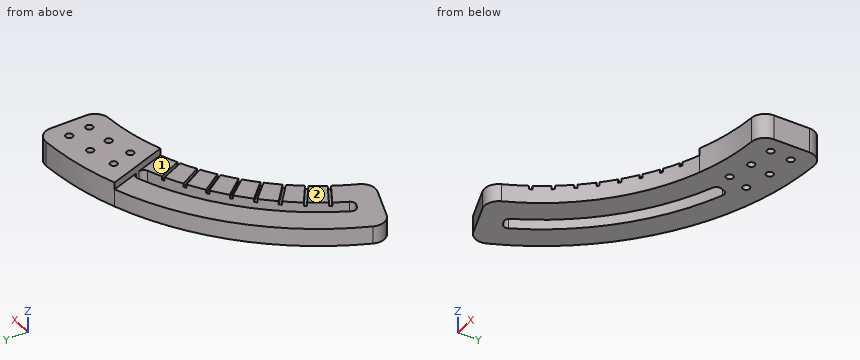
from build123d import *

# Parameters (mm, degrees)
BOSS_EXTRUDE2_DEPTH = 5
SKETCH1_5_R         = 1
BOSS_EXTRUDE3_DEPTH = 7
FILLET1_R           = 1.5
CUT_EXTRUDE1_DEPTH  = 1


with BuildPart() as part:
    # Sketch1 → Boss-Extrude2 (new body)
    with BuildSketch(Plane.XY):
        with BuildLine():
            ThreePointArc((-56.868678478, 24.697234828), (-42.491353844, 45.149583038), (-21.205248886, 58.260942489))
            Line((-21.205248886, 58.260942489), (-23.257369746, 63.899098213))
            Line((-23.257369746, 63.899098213), (-23.599389889, 64.838790834))
            ThreePointArc((-23.599389889, 64.838790834), (-46.615724325, 50.87213624), (-62.535237306, 29.16066006))
            Line((-62.535237306, 29.16066006), (-66.160468454, 30.851133107))
            ThreePointArc((-66.160468454, 30.851133107), (-49.318085156, 53.821245587), (-24.967470463, 68.597561317))
            Line((-24.967470463, 68.597561317), (-25.309490606, 69.537253938))
            Line((-25.309490606, 69.537253938), (-27.361611466, 75.175409663))
            ThreePointArc((-27.361611466, 75.175409663), (-55.059776129, 58.038100009), (-73.631131577, 31.280288725))
            ThreePointArc((-73.631131577, 31.280288725), (-73.618051339, 28.121820986), (-71.317655571, 25.957503806))
            Line((-71.317655571, 25.957503806), (-61.90570605, 22.531834333))
            ThreePointArc((-61.90570605, 22.531834333), (-58.95783549, 22.615790046), (-56.868678478, 24.697234828))
        make_face()
    extrude(amount=BOSS_EXTRUDE2_DEPTH)

    # Sketch1<5> → Boss-Extrude3 (add)
    with BuildSketch(Plane.XY):
        with BuildLine():
            ThreePointArc((-21.205248886, 58.260942489), (-12.61233393, 60.703616308), (-3.757575758, 61.886029315))
            ThreePointArc((-3.757575758, 61.886029315), (-1.087123675, 63.137298701), (0, 65.878676368))
            Line((0, 65.878676368), (0, 75.894663844))
            ThreePointArc((0, 75.894663844), (-1.247011194, 78.796568844), (-4.210526316, 79.889119836))
            ThreePointArc((-4.210526316, 79.889119836), (-15.961038091, 78.39161475), (-27.361611466, 75.175409663))
            Line((-27.361611466, 75.175409663), (-21.205248886, 58.260942489))
        make_face()
        with Locations((-4.594594595, 67.844599641)):
            Circle(SKETCH1_5_R, mode=Mode.SUBTRACT)
        with Locations((-11.808076081, 66.966927205)):
            Circle(SKETCH1_5_R, mode=Mode.SUBTRACT)
        with Locations((-18.886713057, 65.324513545)):
            Circle(SKETCH1_5_R, mode=Mode.SUBTRACT)
        with Locations((-5, 73.830887845)):
            Circle(SKETCH1_5_R, mode=Mode.SUBTRACT)
        with Locations((-12.849965147, 72.875773723)):
            Circle(SKETCH1_5_R, mode=Mode.SUBTRACT)
        with Locations((-20.553187739, 71.088441211)):
            Circle(SKETCH1_5_R, mode=Mode.SUBTRACT)
    extrude(amount=BOSS_EXTRUDE3_DEPTH)

    # Fillet1
    fillet1_edges = [part.edges().sort_by_distance(p)[0] for p in [
        (-66.160468454, 30.851133107, 2.5),
        (-62.535237306, 29.16066006, 2.5),
        (-23.599389889, 64.838790834, 2.5),
        (-24.967470463, 68.597561317, 2.5),
    ]]
    fillet(fillet1_edges, radius=FILLET1_R)

    # Sketch2 → Cut-Extrude1 (cut)
    with BuildSketch(Plane.XY.offset(5)):
        Polygon((-26.182734595, 55.202574904), (-25.457688366, 55.540669514), (-29.670325491, 64.574698983), (-30.395371721, 64.236604373), align=None)
        Polygon((-30.894322803, 52.71053676), (-35.87829712, 61.343033502), (-35.185476797, 61.743033502), (-30.20150248, 53.11053676), align=None)
        Polygon((-35.370786559, 49.817339603), (-41.088167015, 57.982605105), (-40.43284538, 58.441466254), (-34.715464924, 50.276200752), align=None)
        Polygon((-39.578057272, 46.545002412), (-45.985331149, 54.180894073), (-45.372495595, 54.695124161), (-38.965221718, 47.059232499), align=None)
        Polygon((-43.484115072, 42.918429647), (-50.532519147, 49.966833722), (-49.966833722, 50.532519147), (-42.918429647, 43.484115072), align=None)
        Polygon((-47.059232499, 38.965221718), (-54.695124161, 45.372495595), (-54.180894073, 45.985331149), (-46.545002412, 39.578057272), align=None)
        Polygon((-50.276200752, 34.715464924), (-58.441466254, 40.43284538), (-57.982605105, 41.088167015), (-49.817339603, 35.370786559), align=None)
        Polygon((-53.11053676, 30.20150248), (-61.743033502, 35.185476797), (-61.343033502, 35.878297121), (-52.71053676, 30.894322803), align=None)
    extrude(amount=-CUT_EXTRUDE1_DEPTH, mode=Mode.SUBTRACT)


solid = part.part
The model under review builds one solid part; all positions refer to its coordinate system, in mm. Face numbers are marked on the shaded views. A direction names the side the tool comes from. Give positions to 0.01 mm unless a question says otherwise; leave off trailing zeros. Order: outer loops, then holes, each group sorted by start corner. A loop starts at its lowest first (then second) coordinate and runs counter-clockwise, first axis right, second up. Notation, with made-up numbers: M 40.5,62 L 95.5,62 A25 ccw 95.5,88 Z; hole C -37,-12.5 d2. An arc over 180 degrees is marked long. Answer in a Markdown table with one row per item. Add a question column.
1. To check wall thickness, follow line 1 along X through (y, z) = (72, 4.5); line 2 along X through (y, z) = (64.5, 2); line 3 along Z through (x, y) = (-60, 43.5). State the ranges of each line that lie inside material, in increasing order.
2. Add section D-D on x = -66.5. State the section outline as (y, z) points, plus the area to 3 significant figures.
3. Add section B-B on y = 38. State the section outline as (x, z) points, plus the area to 3 significant figures.
4. For pin 1 Ø6 at (x, y) = (-39.5, 49.5) entering from +Z; pin 2 Ø1.6 at (x, y) = (-4.59, 67.84) entering from -Z, all flat-tipped, find the tip position at first contact; note any pin that passes through.
5. Add section A-A on x = -41. State the section outline as (y, z) points.
6. Add section C-C on z = 2.25. State the section outline as (x, y) points, plus the area to 3 significant figures.
7. Machinability: for the marked faces 1 and 2, which of the approach directions +Z, -Z, +X, -X, +Y, -Y give a long, thin tool a straight path to every point of the face, cutting with its end or side? Answer none if there is none.
The answers:
| question | item | result |
|---|---|---|
| 1 | line 1 | -34.87 to -20.96, -20.14 to -13.33, -12.37 to 0 |
| 1 | line 2 | -47.33 to -34.19, -24.64 to -19.45, -18.32 to -0.25 |
| 1 | line 3 | 0 to 5 |
| 2 | outline | M 24.2,0 L 44.47,0 L 44.47,5 L 24.2,5 Z |
| 2 | area | 101 mm2 |
| 3 | outline | M -70.4,0 L -62.33,0 L -62.33,5 L -70.4,5 Z; M -57.59,0 L -48.99,0 L -48.99,5 L -53.57,5 L -53.57,4 L -54.97,4 L -54.97,5 L -57.59,5 Z |
| 3 | area | 82.0 mm2 |
| 4 | pin 1 | z = 5 |
| 4 | pin 2 | through |
| 5 | outline | M 46.51,0 L 55.5,0 L 55.5,5 L 49.48,5 L 49.48,4 L 48.24,4 L 48.24,5 L 46.51,5 Z; M 60.4,0 L 68.69,0 L 68.69,5 L 60.4,5 Z |
| 6 | outline | M -73.63,31.28 A4 ccw -71.32,25.96 L -61.91,22.53 A4 ccw -56.87,24.7 A62 cw -3.76,61.89 A4 ccw 0,65.88 L 0,75.89 A4 ccw -4.21,79.89 A80 ccw Z; hole M -65.5,32.23 A1.5 ccw -64.79,30.21 L -63.88,29.79 A1.5 ccw -61.9,30.48 A69 cw -24.97,64.32 A1.5 ccw -24.11,66.23 L -24.45,67.17 A1.5 ccw -26.4,68.06 A73 ccw Z; hole C -20.55,71.09 d2; hole C -18.89,65.32 d2; hole C -12.85,72.88 d2; hole C -11.81,66.97 d2; hole C -5,73.83 d2; hole C -4.59,67.84 d2 |
| 6 | area | 1,310 mm2 |
| 7 | face 1 | +Z, -X, -Y |
| 7 | face 2 | +Z, +X, -X, +Y, -Y |
